Part print with two shaded views. Sizes in mm from the minimum x, y, z corner. Round coordinates to 2 decimals unless told otherwise and drop trailing zeros. Order: outer loops, then holes, each group sorted by start corner. A loop starts at its lowest first (then second) coordinate and runs counter-clockwise, first axis right, second up. Notation, with made-up numbers: M -12.5,74.25 L 46.5,74.25 A26 ccw 46.5,106.25 Z; hole C -2,75 d2. An arc over 180 degrees is marked long. Answer as a JSON object with one key per item and string values.
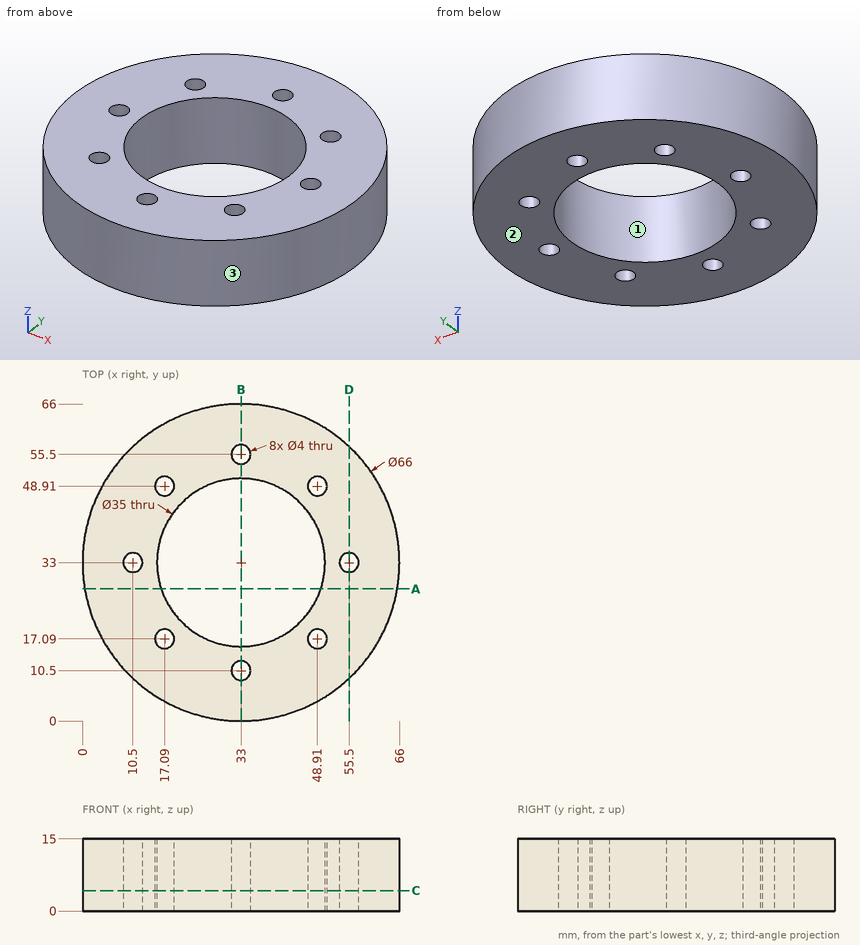
Item 1: Saw through at C-C on z = 4.25. State how many separate pieces and enclosed holes the cut face has, and give its area (3 significant figures).
Worked answers:
{"separate pieces": "1", "enclosed holes": "9", "area": "2,360 mm2"}
Item 2: Wall check: line 1 along Y through (x, z) = (33, 6.5); line 2 along Y through (x, z) = (48.5, 9.5); line 3 along X through (y, z) = (26, 10.5). Give the ranges that are in metal, low to high. Write a range as [from, to].
Worked answers:
{"line 1": "y = [0, 8.5], [12.5, 15.5], [50.5, 53.5], [57.5, 66]", "line 2": "y = [3.87, 15.13], [19.05, 24.88], [41.12, 46.95], [50.87, 62.13]", "line 3": "x = [0.75, 16.96], [49.04, 65.25]"}
Item 3: Saw through at A-A on y = 27.5. List the corners of the cut face in (x, z).
Worked answers:
{"outline": "M 0.46,0 L 16.39,0 L 16.39,15 L 0.46,15 Z; M 49.61,0 L 65.54,0 L 65.54,15 L 49.61,15 Z"}
Item 4: Saw through at D-D on x = 55.5. List the corners of the cut face in (y, z).
Worked answers:
{"outline": "M 8.86,0 L 31,0 L 31,15 L 8.86,15 Z; M 35,0 L 57.14,0 L 57.14,15 L 35,15 Z"}
Item 5: Two-plate mould, pull along Y, no slides. Class the marked faces 1, 2 and 3: released by +Y, released by -Y, zero draft, split by the parting line, or undercut.
Worked answers:
{"face 1": "undercut", "face 2": "zero draft", "face 3": "split by the parting line"}
Item 6: Drop flat-ended pins along their axis: pin 1 Ø4 at (y, z) = (12.5, 5) entering from +X; pin 2 Ø1.5 at (x, z) = (32, 11) entering from -Y; pin 3 Ø5 at (x, z) = (57, 9.5) entering from +Y (3 decimals). Give the stop position or say it passes through.
Worked answers:
{"pin 1": "stops at x = 60.33", "pin 2": "stops at y = 0", "pin 3": "stops at y = 58.035"}
Item 7: Saw through at B-B on x = 33. List the corners of the cut face in (y, z), and give its area (3 significant figures).
Worked answers:
{"outline": "M 0,0 L 8.5,0 L 8.5,15 L 0,15 Z; M 12.5,0 L 15.5,0 L 15.5,15 L 12.5,15 Z; M 50.5,0 L 53.5,0 L 53.5,15 L 50.5,15 Z; M 57.5,0 L 66,0 L 66,15 L 57.5,15 Z", "area": "345 mm2"}
